```python
from build123d import *

# Parameters (mm, degrees)
SKETCH_R  = 5.1
PAD_DEPTH = 6.35


with BuildPart() as part:
    # Sketch → Pad (new body)
    with BuildSketch(Plane.XY):
        with BuildLine():
            ThreePointArc((-27.5, 12.5), (-40, 1e-06), (-27.500002, -12.5))
            Line((27.499963, -12.5), (-27.500002, -12.5))
            ThreePointArc((27.499963, -12.5), (39.999963, -1.8e-05), (27.5, 12.5))
            Line((-27.5, 12.5), (27.5, 12.5))
        make_face()
        with Locations((-27.5, 0)):
            Circle(SKETCH_R, mode=Mode.SUBTRACT)
        with Locations((27.499963, 0)):
            Circle(SKETCH_R, mode=Mode.SUBTRACT)
    extrude(amount=PAD_DEPTH)


solid = part.part
```
Part model, mm, in its own coordinate system. Round coordinates to 2 decimals unless told otherwise and drop trailing zeros. Loops run counter-clockwise (first coordinate to the right, second up) from the corner with the lowest first, then second, coordinate; pieces in that order, holes last. Notation, with made-up numbers: (44.25, 35.5) -> (92.25, 35.5) arc R10 ccw to (92.25, 43.5) -> close; hole circle Ø11 at (-20.5, 8). An arc over 180 degrees is marked (long way). Use CSV: the item, a comma, the result in double quotes. Start each with the question number.
1) Cut at C-C, the plane x = -35. Write the cut outline in (y, z), plus the area to 3 significant figures.
2) Pull direction X, two halves, no side cores. Call faces 1 (the flat face through (0, 12.5, 3)), 2 (the cylindrical face through (-40, 0, 3)), 3 (the cylindrical face through (32.364, 1.532, 3.131)): +X half, -X half, draft (parallel to the pull), parting line (faces both ways), or undercut.
3) Cut at A-A, the plane y = 0. Write the cut outline in (x, z), plus the area to 3 significant figures.
4) Drop a flat-ended pin along its axis: P1, Ø1, axis at y = 1, z = 4, coming from the -X side. Give the stop position or say it passes through.
5) Wall check: L1, parallel to Y at x = -27.5, z = 2; L2, parallel to X at y = -0.25, z = 5.75; L3, parallel to Y at x = 31, z = 5.75. Give the ranges that are in metal, low to high. Write a range as [from, to].
6) Cut at B-B, the plane z = 3.5. Write the cut outline in (x, y), plus the area to 3 significant figures.
Determined:
1,outline,"(-10, 0) -> (10, 0) -> (10, 6.35) -> (-10, 6.35) -> close"
1,area,"127 mm2"
2,face 1,"draft"
2,face 2,"-X half"
2,face 3,"undercut"
3,outline,"(-40, 0) -> (-32.6, 0) -> (-32.6, 6.35) -> (-40, 6.35) -> close; (-22.4, 0) -> (22.4, 0) -> (22.4, 6.35) -> (-22.4, 6.35) -> close; (32.6, 0) -> (40, 0) -> (40, 6.35) -> (32.6, 6.35) -> close"
3,area,"378 mm2"
4,P1,"stops at x = -39.99"
5,L1,"y = [-12.5, -5.1], [5.1, 12.5]"
5,L2,"x = [-40, -32.59], [-22.41, 22.41], [32.59, 40]"
5,L3,"y = [-12, -3.71], [3.71, 12]"
6,outline,"(-27.5, -12.5) -> (27.5, -12.5) arc R12.5 ccw to (27.5, 12.5) -> (-27.5, 12.5) arc R12.5 ccw to start; hole circle Ø10.2 at (-27.5, 0); hole circle Ø10.2 at (27.5, 0)"
6,area,"1,700 mm2"
